Geometry: see drawing. Coordinates: mm, zero at the bounding-box minimum. Coordinates: 2 decimals unless noted, no trailing zeros. Loops run counter-clockwise (first coordinate to the right, second up) from the corner with the lowest first, then second, coordinate; pieces in that order, holes last. Notation, with made-up numbers: (74, -27) - (102, -27) arc R22 ccw to (102, 1) - close; hole circle Ø10 at (86.25, 89). An arc over 180 degrees is marked (long way). Use one line per item in the form item = value.
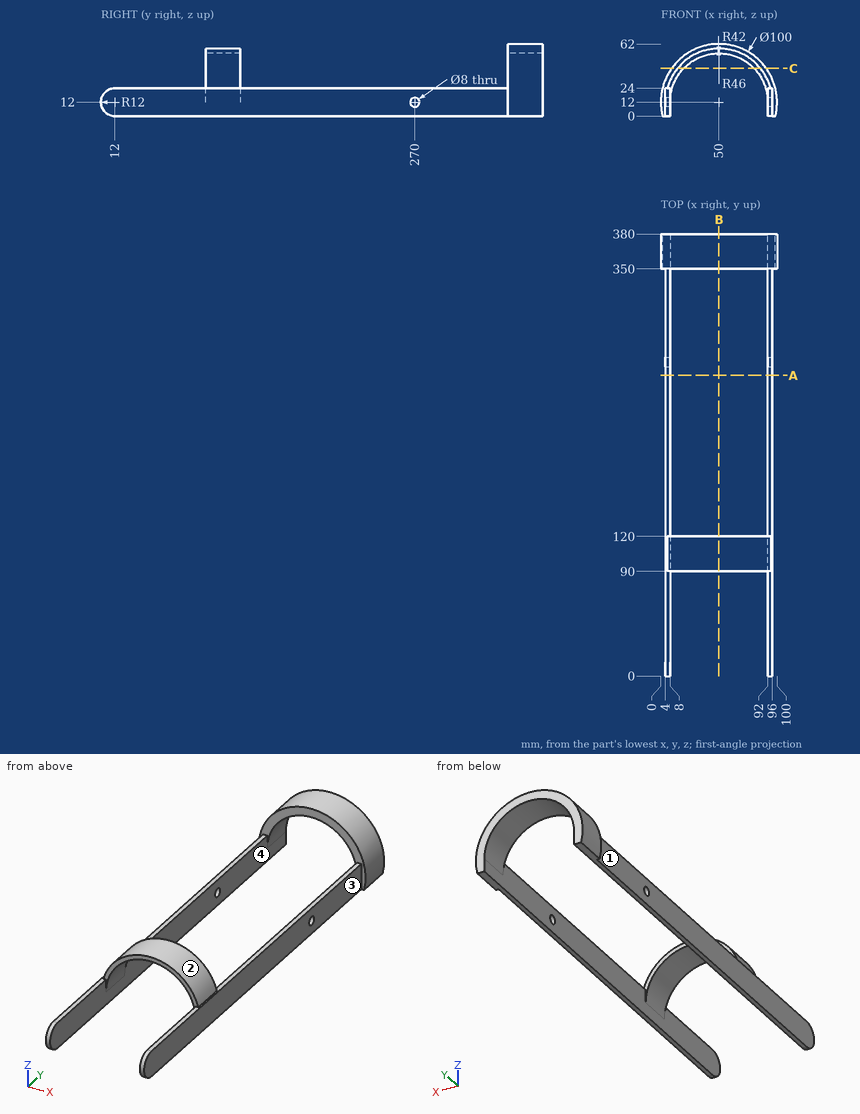
Q1. Pull-direction query (X, two-part tool) for the marked faces 1, 2, 3 and 4; classes: pulls with the +X half, pulls with the -X half, needs draft (parallel to the pull), parting line crosses it, or undercut.
Check values:
face_1 = pulls with the -X half
face_2 = parting line crosses it
face_3 = pulls with the +X half
face_4 = undercut
Q2. Cut plane B-B, the plane x = 50. Return loops of the section in (y, z), then the cut area to 3 significant figures.
Check values:
outline = (90, 54) - (120, 54) - (120, 58) - (90, 58) - close; (350, 54) - (380, 54) - (380, 62) - (350, 62) - close
area = 360 mm²
Q3. Ray query, line 1 along Z through (x, y) = (5.3, 270); line 2 along Y through (x, z) = (93, 12); line 3 along X through (y, z) = (208, 23). Return the intervals inside material, ascending. Write a range as [from, to].
Check values:
line_1 = [0, 8], [16, 24]
line_2 = [0, 266], [274, 380]
line_3 = [4, 8], [92, 96]
Q4. Cut plane C-C, the plane z = 41. Return loops of the section in (x, y), then the cut area to 3 significant figures.
Check values:
outline = (9.27, 350) - (19.62, 350) - (19.62, 380) - (9.27, 380) - close; (14.29, 90) - (19.62, 90) - (19.62, 120) - (14.29, 120) - close; (80.38, 90) - (85.71, 90) - (85.71, 120) - (80.38, 120) - close; (80.38, 350) - (90.73, 350) - (90.73, 380) - (80.38, 380) - close
area = 941 mm²
Q5. Cut plane A-A, the plane y = 258.5. Return loops of the section in (x, z), then the cut area to 3 significant figures.
Check values:
outline = (4, 0) - (8, 0) - (8, 24) - (4, 24) - close; (92, 0) - (96, 0) - (96, 24) - (92, 24) - close
area = 192 mm²
Q6. First-contact query: P1, Ø2, axis at x = 6.5, y = 227.5, coming from the +Z side; P2, Ø7, axis at y = 147, z = 15.5, coming from the -X side; P3, Ø2, axis at y = 215.5, z = 24, coming from the +X side. Flat tips, straight axial feed; report the tip coordinate or a pass-through.
Check values:
P1 = 24
P2 = 4
P3 = 96
